Geometry check sheet. Reference: the model listing, model coordinates, mm. Face numbers are marked on the shaded views. A direction names the side the tool comes from. Give positions to 0.01 mm unless a question says otherwise; leave off trailing zeros. Loops run counter-clockwise (first coordinate to the right, second up) from the corner with the lowest first, then second, coordinate; pieces in that order, holes last. Notation, with made-up numbers: (22.25, -9.5) -> (54.25, -9.5) arc R26 cw to (54.25, 13.5) -> close; hole circle Ø6 at (66, 34.25). An arc over 180 degrees is marked (long way). Answer in a Markdown table with one row per item. Add a question column.
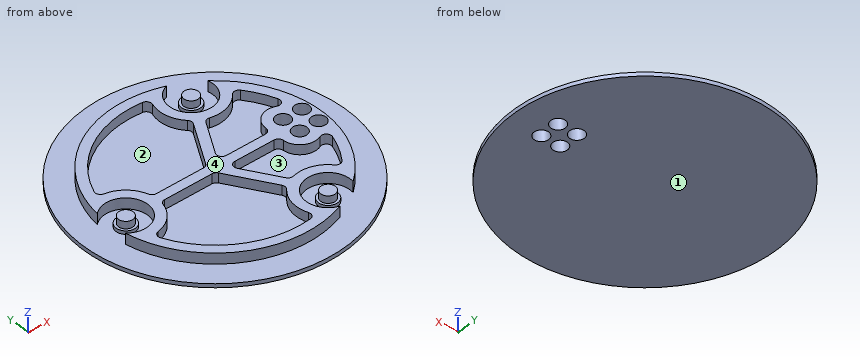
Autodesk Inventor part; units mm, degrees
ref_plane "YZ Plane" through (0, 0, 0) normal (1, 0, 0) x (0, 1, 0)
ref_plane "XZ Plane" through (0, 0, 0) normal (0, 1, 0) x (-1, 0, 0)
ref_plane "XY Plane" through (0, 0, 0) normal (0, 0, 1) x (1, 0, 0)
sketch "スケッチ1" plane through (0, 0, 0) normal (0, 0, 1) x (1, 0, 0)
  circle A0 centre (-18, 0) radius 27
  line L0 (0, 0) -> (-18, 0) construction
  circle A1 centre (-36.7, 0) radius 1.5
  circle A2 centre (-36.7, 0) radius 4 construction
  circle A3 centre (-36.7, 0) radius 4.5
  circle A4 centre (-8.65, -16.1947) radius 4.5
  circle A5 centre (-8.65, -16.1947) radius 4 construction
  circle A6 centre (-8.65, -16.1947) radius 1.5
  circle A7 centre (-8.65, 16.1947) radius 4.5
  circle A8 centre (-8.65, 16.1947) radius 4 construction
  circle A9 centre (-8.65, 16.1947) radius 1.5
  circle A10 centre (-18, 0) radius 22
  line L1 (-36.7, 0) -> (-18, 0) construction
  circle A11 centre (-18, 0) radius 22.7 construction
  circle A12 centre (-36.7, 0) radius 2
  circle A13 centre (-8.65, -16.1947) radius 2
  circle A14 centre (-8.65, 16.1947) radius 2
  circle A15 centre (-1.9799, 1.9799) radius 2.8
  circle A16 centre (-1.9799, 1.9799) radius 1.5
  circle A17 centre (-1.9799, -1.9799) radius 1.5
  circle A18 centre (-1.9799, -1.9799) radius 2.8
  circle A19 centre (1.9799, -1.9799) radius 1.5
  circle A20 centre (1.9799, -1.9799) radius 2.8
  circle A21 centre (1.9799, 1.9799) radius 1.5
  circle A22 centre (1.9799, 1.9799) radius 2.8
  line L2 (0, 0) -> (-1.9799, 1.9799)
  point P0 (-1.5877, 1.6905)
  point P1 (-5.0591, 12.5113)
  point P2 (1.2886, 2.8639)
  point P3 (1.2886, -2.8639)
  point P4 (-5.0591, -12.5113)
  point P5 (-13.6354, -17.4628)
  point P6 (-35.3056, -4.9515)
  point P7 (-35.3056, 4.9515)
  point P8 (-13.6354, 17.4628)
  point P9 (0.5827, -2.75)
  point P10 (-4.16, 16.8432)
  point P11 (-4.16, -16.8432)
  point P12 (-10.3333, -20.4074)
  point P13 (-39.5067, -3.5642)
  point P14 (-39.5067, 3.5642)
  point P15 (-10.3333, 20.4074)
  point P16 (-0.2113, 2.75)
  point P17 (-35.9375, 1.4987)
  point P18 (-35.9375, -1.4987)
  point P19 (-7.7333, -14.785)
  point P20 (-10.3292, -16.2837)
  point P21 (-10.3292, 16.2837)
  point P22 (-7.7333, 14.785)
  point P23 (4, 0.041)
  point P24 (4, -0.041)
  point P25 (3.5801, -4.2776)
  point P26 (-4.2595, -17.1813)
  point P27 (-9.9908, -20.4903)
  point P28 (-39.7497, -3.3089)
  point P29 (-39.7497, 3.3089)
  point P30 (-9.9908, 20.4903)
  point P31 (-4.2595, 17.1813)
  point P32 (3.5801, 4.2776)
  dimension "d10" = 54
  dimension "d13" = 3
  dimension "d14" = 8
  dimension "d15" = 9
  dimension "d16" = 360
  dimension "d19" = 5
  dimension "d23" = 4
  dimension "d24" = 360
  dimension "d25" = 5.6
  dimension "d26" = 3
  dimension "d30" = 360
  dimension "d46" = 45
  dimension "d47" = 18
  dimension "d49" = 44
  dimension "d50" = 18.7
  dimension "d53" = 0.7
extrude "押し出し1" add sketch "スケッチ1" along normal blind 0.8 contours A0 | A3 A10 | A10 A3 | A10 A7 | A7 A10 | A10 A4 | A4 A10 | A22 A10 | A10 A20
extrude "押し出し2" add sketch "スケッチ1" along normal blind 1.5 contours A12 | A13 | A14
extrude "押し出し3" add sketch "スケッチ1" along normal blind 3 contours A1 | A3 A10 A7 A22 A15 A18 A20 A4 | A10 A22 A20 A21 A15 | A20 A18 A19 A22 A10 | A10 A20 A22 | A22 A16 A18 A15 | A15 A21 A22 A16 | A20 A17 A18 A19 | A18 A15 A17 A20 | A22 A19 A20 A21 | A18 A16 A15 A17 | A21 A20 A15 | A22 L2 A16 | A18 A22 A19 | A17 A15 A20 | A18 A16 L2 | A6 | A9 picked at (0.5491, 0.5309) picked at (0.5491, -0.5309) picked at (-0.5491, -0.5309)
sketch "スケッチ2" plane through (0, 0, 3) normal (0, 0, 1) x (1, 0, 0)
  arc A0 (-39.7497, -3.3089) -> (-39.7497, 3.3089) centre (-36.7, 0) ccw
  arc A1 (-39.7497, -3.3089) -> (-9.9908, -20.4903) centre (-18, 0) ccw
  arc A2 (-4.2595, -17.1813) -> (-9.9908, -20.4903) centre (-8.65, -16.1947) ccw
  arc A3 (-4.2595, -17.1813) -> (-4.2595, 17.1813) centre (-18, 0) ccw
  arc A4 (-9.9908, 20.4903) -> (-4.2595, 17.1813) centre (-8.65, 16.1947) ccw
  arc A5 (-9.9908, 20.4903) -> (-39.7497, 3.3089) centre (-18, 0) ccw
  circle A6 centre (1.9799, 1.9799) radius 1.5
  circle A7 centre (-1.9799, -1.9799) radius 1.5
  circle A8 centre (-1.9799, 1.9799) radius 1.5
  circle A9 centre (1.9799, -1.9799) radius 1.5
  arc A10 (-36.9155, -6.4964) -> (-36.9155, 6.4964) centre (-36.7, 0) ccw
  arc A11 (-36.9155, -6.4964) -> (-14.1683, -19.6295) centre (-18, 0) ccw
  arc A12 (-2.9162, -13.1331) -> (-14.1683, -19.6295) centre (-8.65, -16.1947) ccw
  arc A13 (-2.9162, -13.1331) -> (-2.9162, 13.1331) centre (-18, 0) ccw
  arc A14 (-14.1683, 19.6295) -> (-2.9162, 13.1331) centre (-8.65, 16.1947) ccw
  arc A15 (-14.1683, 19.6295) -> (-36.9155, 6.4964) centre (-18, 0) ccw
  circle A16 centre (-1.9799, 1.9799) radius 3.5
  circle A17 centre (-1.9799, -1.9799) radius 3.5
  line L0 (-36.7, 0) -> (0, 0) construction
  line L1 (-36.7, -1) -> (0, -1)
  line L2 (0, 1) -> (-36.7, 1)
  arc A18 (-36.7, 1) -> (-36.7, -1) centre (-36.7, 0) ccw
  arc A19 (0, -1) -> (0, 1) centre (0, 0) ccw
  line L3 (-8.65, 16.1947) -> (-18.35, 0) construction
  line L4 (-9.5079, 16.7085) -> (-19.2079, 0.5138)
  line L5 (-17.4921, -0.5138) -> (-7.7921, 15.6808)
  arc A20 (-7.7921, 15.6808) -> (-9.5079, 16.7085) centre (-8.65, 16.1947) ccw
  arc A21 (-19.2079, 0.5138) -> (-17.4921, -0.5138) centre (-18.35, 0) ccw
  line L6 (-18.35, 0) -> (-8.65, -16.1947) construction
  line L7 (-19.2079, -0.5138) -> (-9.5079, -16.7085)
  line L8 (-7.7921, -15.6808) -> (-17.4921, 0.5138)
  arc A22 (-17.4921, 0.5138) -> (-19.2079, -0.5138) centre (-18.35, 0) ccw
  arc A23 (-9.5079, -16.7085) -> (-7.7921, -15.6808) centre (-8.65, -16.1947) ccw
  circle A24 centre (-0.0604, 6.1052) radius 1.05
  circle A25 centre (-0.0604, -6.1052) radius 1.05
  point P0 (-13.5, 8.0973)
  point P1 (-13.5, -8.0973)
  point P2 (0.9336, -6.4435)
  point P3 (-0.5034, -5.1532)
  point P4 (-5.3399, -1)
  point P5 (-16.5854, -1)
  point P6 (-11.0923, -10.171)
  point P7 (-0.5034, 5.1532)
  point P8 (0.9336, 6.4435)
  point P9 (-11.0923, 10.171)
  point P10 (-16.5854, 1)
  point P11 (-5.3399, 1)
  point P12 (-12.8081, -11.1986)
  point P13 (-18.9167, -1)
  point P14 (-30.2774, -1)
  point P15 (-30.2774, 1)
  point P16 (-18.9167, 1)
  point P17 (-12.8081, 11.1986)
  dimension "d58" = 2
  dimension "d59" = 2
  dimension "d60" = 2
  dimension "d61" = 2
  dimension "d62" = 2
  dimension "d63" = 2
  dimension "d64" = 2.1
  dimension "d65" = 2.1
extrude "押し出し4" cut sketch "スケッチ2" against normal blind 2 contours L1 L7 A12 A11 A10 | A10 A15 A14 L4 L2 | L8 L1 A17 A25 A13 A12 | L5 A14 A13 A24 A16 L2 | A25 | A24
fillet "フィレット1" radius 1.05 18 edges at (-30.2774, 1, 2) (-36.9155, 6.4964, 2) (-14.1683, 19.6295, 2) (-12.8081, 11.1986, 2) (-18.9167, 1, 2) (-18.9167, -1, 2) (-30.2774, -1, 2) (-36.9155, -6.4964, 2) (-14.1683, -19.6295, 2) (-12.8081, -11.1986, 2) (-2.9162, -13.1331, 2) (-11.0923, -10.171, 2) (-16.5854, -1, 2) (-5.3399, 1, 2) (-5.3399, -1, 2) (-11.0923, 10.171, 2) (-2.9162, 13.1331, 2) (-16.5854, 1, 2)
properties part number "クランク3t" material "ポリカーボネート、スモーク"
1. Access from +Z, -Z, +X, -X, +Y, -Y to the whole of each face (thin tool, end or side, straight path). Record for the marked faces 1 and 2.
2. Release check for a two-part mould opening along Y. For the marked faces 3 and 4 record: released by +Y, released by -Y, zero draft, split by the parting line, or undercut.
3. Sectioned sample at C-C (z = 2). Count the separate pieces of the cut face and the enclosed holes in it, plus the area to 3 significant figures.
4. Material ranges on L1, parallel to X at y = -8.5, z = 1.35; L2, parallel to X at y = 7, z = 2.6; L3, parallel to X at y = 2, z = 2.35, recorded low to high. Write a range as from..to.
5. Sectioned sample at A-A (x = -22.5). Enter the section's corners in (y, z), plus the area to 3 significant figures.
6. Sectioned sample at B-B (y = -13.5). Enter the section's corners in (x, z).
7. Gauge pin test, flat ends, axial feed: pin 1 Ø0.6 at (x, z) = (-9, 2) entering from +Y; pin 2 Ø1 at (x, z) = (-28, 2.5) entering from +Y; pin 3 Ø1.6 at (x, z) = (-10, 2.5) entering from -Y. Record the tip position at first contact, or that the pin passes through.
Response:
| question | item | result |
|---|---|---|
| 1 | face 1 | -Z, +X, -X, +Y, -Y |
| 1 | face 2 | +Z |
| 2 | face 3 | undercut |
| 2 | face 4 | zero draft |
| 3 | separate pieces | 4 |
| 3 | enclosed holes | 8 |
| 3 | area | 491 mm2 |
| 4 | L1 | x = -38.29..-36.1, -14.42..-12.09, 0.1..2.29 |
| 4 | L2 | x = -38.86..-36.38, -15.32..-12.99, 0.73..2.86 |
| 4 | L3 | x = -32.67..-30.52, -18.32..-15.78, -5.48..-3.48, -0.48..0.48, 3.48..3.91 |
| 5 | outline | (-26.62, 0) -> (26.62, 0) -> (26.62, 0.8) -> (21.53, 0.8) -> (21.53, 3) -> (19.49, 3) -> (19.49, 1) -> (1, 1) -> (1, 3) -> (-1, 3) -> (-1, 1) -> (-19.49, 1) -> (-19.49, 3) -> (-21.53, 3) -> (-21.53, 0.8) -> (-26.62, 0.8) -> close |
| 5 | area | 63.4 mm2 |
| 6 | outline | (-41.38, 0) -> (5.38, 0) -> (5.38, 0.8) -> (-0.63, 0.8) -> (-0.63, 3) -> (-5.05, 3) -> (-5.05, 0.8) -> (-12.25, 0.8) -> (-12.25, 3) -> (-14.57, 3) -> (-14.57, 1) -> (-32.76, 1) -> (-32.76, 3) -> (-35.37, 3) -> (-35.37, 0.8) -> (-41.38, 0.8) -> close |
| 7 | pin 1 | stops at y = 17.69 |
| 7 | pin 2 | stops at y = 19.84 |
| 7 | pin 3 | stops at y = -20.79 |
